Part model, mm, in its own coordinate system. A direction names the side the tool comes from. Coordinates: 2 decimals unless noted, no trailing zeros. Loops run counter-clockwise (first coordinate to the right, second up) from the corner with the lowest first, then second, coordinate; pieces in that order, holes last. Notation, with made-up numbers: M 34,62.5 L 54,62.5 A12 cw 54,68.5 Z; hole C 71.5,81 d7. An arc over 180 degrees is marked long. Use CSV: the item, a comma, the result in double quotes. Start each with the question number.
from build123d import *

# Parameters (mm, degrees)
SKETCH_4_R           = 10
EXTRUDE_2_DEPTH      = 2.5
SKETCH_6_R           = 1.5
CUT_EXTRUDE_9_DEPTH  = 2.5
SKETCH_7_R           = 4.4
EXTRUDE_3_DEPTH      = 2
SKETCH_8_R           = 3
CUT_EXTRUDE_10_DEPTH = 3


with BuildPart() as part:
    # Sketch 4 → Extrude 2 (new body)
    with BuildSketch(Plane(origin=(0, 0, 0), x_dir=(1, 0, 0), z_dir=(0, 1, 0))):
        with Locations(Location((0, 0, 0), (0, 0, 270))):
            Circle(SKETCH_4_R)
    extrude(amount=EXTRUDE_2_DEPTH)

    # Sketch 6 → Cut-Extrude 9 (cut)
    with BuildSketch(Plane(origin=(0, 2.5, 0), x_dir=(1, 0, 0), z_dir=(0, 1, 0))):
        with Locations(Location((0, 7, 0), (0, 0, 270))):
            Circle(SKETCH_6_R)
        with Locations(Location((0, 0, 0), (0, 0, 270))):
            Circle(SKETCH_6_R)
        with Locations(Location((7, 0, 0), (0, 0, 270))):
            Circle(SKETCH_6_R)
        with Locations(Location((-7, 0, 0), (0, 0, 270))):
            Circle(SKETCH_6_R)
        with Locations(Location((0, -7, 0), (0, 0, 270))):
            Circle(SKETCH_6_R)
    extrude(amount=-CUT_EXTRUDE_9_DEPTH, mode=Mode.SUBTRACT)

    # Sketch 7 → Extrude 3 (add)
    with BuildSketch(Plane(origin=(0, 2.5, 0), x_dir=(1, 0, 0), z_dir=(0, 1, 0))):
        with Locations(Location((0, 0, 0), (0, 0, 270))):
            Circle(SKETCH_7_R)
    extrude(amount=EXTRUDE_3_DEPTH)

    # Sketch 8 → Cut-Extrude 10 (cut)
    with BuildSketch(Plane(origin=(0, 4.5, 0), x_dir=(1, 0, 0), z_dir=(0, 1, 0))):
        with Locations(Location((0, 0, 0), (0, 0, 270))):
            Circle(SKETCH_8_R)
    extrude(amount=-CUT_EXTRUDE_10_DEPTH, mode=Mode.SUBTRACT)


solid = part.part
1. Two-plate mould, pull along Z, no slides. Class faces 3 (the face through (0.9, 3.02, 2.86)), 4 (the face through (-9.76, 1.23, -2.17)), 5 (the face through (-3, 4.5, 1)): pulls with the +Z half, pulls with the -Z half, needs draft (parallel to the pull), parting line crosses it, or undercut.
2. Tool access for faces 1 (the face through (0.45, 0.76, 1.43)), 2 (the face through (4.363, 3.486, -0.573)): list every direction of +Z, -Z, +X, -X, +Y, -Y with a clear straight run to the whole face (end or side of a thin tool).
3. Slice it at B-B, the plane z = 0. List the corners of the cut face in (x, y).
4. Wall check: probe 1 along X at (y, z) = (1.85, 0); probe 2 along X at (y, z) = (0.75, 0); probe 3 along X at (y, z) = (3.2, 0). Give the ranges that are in metal, low to high.
5. Slice it at A-A, the plane x = 0. List the corners of the cut face in (y, z).
6. Slice it at D-D, the plane x = -7. List the corners of the cut face in (y, z), and give its area (3 significant figures).
7. Slice it at C-C, the plane y = 2.2. List the corners of the cut face in (x, z), and give its area (3 significant figures).
8. Pin check, flat tips, straight feed: pin 1 (2.5 mm diameter, centred on x = 7, z = 0, fed in from +Y); pin 2 (1 mm diameter, centred on x = 5.5, z = -5.5, fed in from +Y); pin 3 (3.5 mm diameter, centred on x = 0, z = 0, fed in from +Y). Stop position of each tip, or through.
Found:
1,face 3,"undercut"
1,face 4,"parting line crosses it"
1,face 5,"needs draft"
2,face 1,"+Y, -Y"
2,face 2,"+Y"
3,outline,"M -10,0 L -8.5,0 L -8.5,2.5 L -10,2.5 Z; M -5.5,0 L -1.5,0 L -1.5,1.5 L -3,1.5 L -3,4.5 L -4.4,4.5 L -4.4,2.5 L -5.5,2.5 Z; M 1.5,0 L 5.5,0 L 5.5,2.5 L 4.4,2.5 L 4.4,4.5 L 3,4.5 L 3,1.5 L 1.5,1.5 Z; M 8.5,0 L 10,0 L 10,2.5 L 8.5,2.5 Z"
4,probe 1,"-10 to -8.5, -5.5 to -3, 3 to 5.5, 8.5 to 10"
4,probe 2,"-10 to -8.5, -5.5 to -1.5, 1.5 to 5.5, 8.5 to 10"
4,probe 3,"-4.4 to -3, 3 to 4.4"
5,outline,"M 0,-10 L 2.5,-10 L 2.5,-8.5 L 0,-8.5 Z; M 0,-5.5 L 2.5,-5.5 L 2.5,-4.4 L 4.5,-4.4 L 4.5,-3 L 1.5,-3 L 1.5,-1.5 L 0,-1.5 Z; M 0,1.5 L 1.5,1.5 L 1.5,3 L 4.5,3 L 4.5,4.4 L 2.5,4.4 L 2.5,5.5 L 0,5.5 Z; M 0,8.5 L 2.5,8.5 L 2.5,10 L 0,10 Z"
6,outline,"M 0,-7.14 L 2.5,-7.14 L 2.5,-1.5 L 0,-1.5 Z; M 0,1.5 L 2.5,1.5 L 2.5,7.14 L 0,7.14 Z"
6,area,"28.2 mm^2"
7,outline,"C 0,0 d20; hole C -7,0 d3; hole C 0,0 d6; hole C 0,-7 d3; hole C 0,7 d3; hole C 7,0 d3"
7,area,"258 mm^2"
8,pin 1,"through"
8,pin 2,"y = 2.5"
8,pin 3,"y = 1.5"
